Could you check a few things on this model? Use its own coordinates, in mm. A direction names the side the tool comes from. Give positions to 0.01 mm unless a question says otherwise; leave off trailing zeros. Order: outer loops, then holes, each group sorted by start corner. A loop starts at its lowest first (then second) coordinate and runs counter-clockwise, first axis right, second up.
(1) If we mould it in two halves opening along Z, with no side actions, what happens to faces 1 (the flat face through (0, -1, 20)), 2 (the flat face through (10, -1, 9)), 3 (the cylindrical face through (-9, 0, 6))? For each: released by +Z, released by -Z, zero draft, split by the parting line, or undercut.
(2) Imagine slicing it at C-C, the plane y = 0. Write out the boundary of the cut face in (x, z).
(3) If I drill on probe 1 along Z at (x, y) = (8.85, 0); probe 2 along Z at (x, y) = (-5.25, 20.5); probe 3 along X at (y, z) = (50, 10), over which ranges is the centre line in solid material (lowest first)?
(4) Imagine slicing it at A-A, the plane z = 15. Write out the boundary of the cut face in (x, y).
(5) Imagine slicing it at D-D, the plane z = 0. Write out the boundary of the cut face in (x, y), then the cut area to 3 significant figures.
(6) Will these pins go through, and if not, where does the flat tip stop? pin 1 (14 mm diameter, centred on y = 0, z = 0, fed in from -X); pin 2 (12 mm diameter, centred on x = 3.5, z = -2, fed in from -Y).
(7) On a 3-axis mill with a long thin cutter (end or side, diameter ignored), from which of +Z, -Z, +X, -X, +Y, -Y can I reach the whole of each face in a straight line? I mean faces 4 (the flat face through (-10, -1, -9)), 5 (the flat face through (0, -1, -18.4)). Say none if no direction works.
(8) Imagine slicing it at B-B, the plane x = 1.25. Write out the boundary of the cut face in (y, z).
Autodesk Inventor part; units mm, degrees
ref_plane "YZ Plane" through (0, 0, 0) normal (1, 0, 0) x (0, 1, 0)
ref_plane "XZ Plane" through (0, 0, 0) normal (0, 1, 0) x (-1, 0, 0)
ref_plane "XY Plane" through (0, 0, 0) normal (0, 0, 1) x (1, 0, 0)
sketch "スケッチ2" plane through (0, 0, 0) normal (0, 1, 0) x (-1, 0, 0)
  line L0 (10, -20) -> (-10, -20)
  line L1 (-10, -20) -> (-10, 20)
  line L2 (-10, 20) -> (10, 20)
  line L3 (10, 20) -> (10, -20)
  line L4 (10, -20) -> (-10, 20) construction
  line L5 (-10, -20) -> (10, 20) construction
  line L6 (8.4, 18.4) -> (-8.4, 18.4)
  line L7 (-8.4, 18.4) -> (-8.4, -18.4)
  line L8 (-8.4, -18.4) -> (8.4, -18.4)
  line L9 (8.4, -18.4) -> (8.4, 18.4)
  point P0 (0, 0)
  dimension "d7" = 20
  dimension "d8" = 40
  dimension "d9" = 1.6
extrude "押し出し2" add sketch "スケッチ2" along normal mid plane 150
sketch "スケッチ5" plane through (10, -75, -20) normal (1, 0, 0) x (0, 0, -1)
  point P0 (-20, 75)
  point P1 (-20, 75)
hole "穴2" at (10, 0, 0) direction (-1, 0, 0) diameter 12 end through all
chamfer "面取り1" distance 20 angle 45 2 edges at (10, -75, 0) (10, 75, 0)
properties part number "Pipe3"
Answer block:
1. face 1: released by +Z
1. face 2: zero draft
1. face 3: undercut
2. outline: (-10, -20) - (10, -20) - (10, -6) - (8.4, -6) - (8.4, -18.4) - (-8.4, -18.4) - (-8.4, -6) - (-10, -6) - close; (-10, 6) - (-8.4, 6) - (-8.4, 18.4) - (8.4, 18.4) - (8.4, 6) - (10, 6) - (10, 20) - (-10, 20) - close
3. probe 1: z = -20 to -6, 6 to 20
3. probe 2: z = -20 to -18.4, 18.4 to 20
3. probe 3: x = -10 to -8.4, 8.4 to 10
4. outline: (-10, -75) - (-8.4, -73.4) - (-8.4, 73.4) - (-10, 75) - close; (8.4, -56.6) - (10, -55) - (10, 55) - (8.4, 56.6) - close
5. outline: (-10, -75) - (-8.4, -73.4) - (-8.4, -6) - (-10, -6) - close; (-10, 6) - (-8.4, 6) - (-8.4, 73.4) - (-10, 75) - close; (8.4, -56.6) - (10, -55) - (10, -6) - (8.4, -6) - close; (8.4, 6) - (10, 6) - (10, 55) - (8.4, 56.6) - close
5. area: 378 mm2
6. pin 1: stops at x = -10
6. pin 2: stops at y = -56.6
7. face 4: +Z, -Z, -X, +Y, -Y
7. face 5: +Y, -Y
8. outline: (-63.75, -20) - (63.75, -20) - (63.75, -18.4) - (-63.75, -18.4) - close; (-63.75, 18.4) - (63.75, 18.4) - (63.75, 20) - (-63.75, 20) - close
